```python
from build123d import *

# Parameters (mm, degrees)
F1_DEPTH = 1


with BuildPart() as f1:
    # F0 (on Front) → F1 (new body)
    with BuildSketch(Plane.XZ):
        with BuildLine():
            ThreePointArc((-19.4142135624, 19.4142135624), (-19.847759065, 18.7653668647), (-20, 18))
            Line((-20, 18), (-20, 5))
            ThreePointArc((-20, 5), (-19.7071067812, 4.2928932188), (-19, 4))
            Line((-19, 4), (-16.5, 4))
            ThreePointArc((-16.5, 4), (-15.7928932188, 4.2928932188), (-15.5, 5))
            Line((-15.5, 5), (-15.5, 7))
            ThreePointArc((-15.5, 7), (-15.7928932188, 7.7071067812), (-16.5, 8))
            ThreePointArc((-16.5, 8), (-16.8535533906, 8.1464466094), (-17, 8.5))
            ThreePointArc((-17, 8.5), (-16.4142135624, 9.9142135624), (-15, 10.5))
            Line((-15, 10.5), (-13.0961940777, 10.5))
            ThreePointArc((-13.0961940777, 10.5), (-12.330827213, 10.347759065), (-11.6819805153, 9.9142135624))
            Line((-11.6819805153, 9.9142135624), (-8.3357864376, 6.5680194847))
            ThreePointArc((-8.3357864376, 6.5680194847), (-7.902240935, 5.919172787), (-7.75, 5.1538059223))
            Line((-7.75, 5.1538059223), (-7.75, 0))
            Line((-7.75, 0), (-3.4, 0))
            ThreePointArc((-3.4, 0), (-3.1411904105, 1.30112367), (-2.404163056, 2.404163056))
            Line((-2.404163056, 2.404163056), (-12.2464466094, 12.2464466094))
            ThreePointArc((-12.2464466094, 12.2464466094), (-12.4086582838, 12.1380602337), (-12.6, 12.1))
            Line((-12.6, 12.1), (-17.7, 12.1))
            ThreePointArc((-17.7, 12.1), (-18.0535533906, 12.2464466094), (-18.2, 12.6))
            Line((-18.2, 12.6), (-18.2, 17.2))
            ThreePointArc((-18.2, 17.2), (-18.1238795325, 17.5826834324), (-17.9071067812, 17.9071067812))
            Line((-17.9071067812, 17.9071067812), (-19.4142135624, 19.4142135624))
        make_face()
    extrude(amount=F1_DEPTH)

    # F2: F1 across face


with BuildPart() as f1_1:
    add(f1.part)
    add(f1.part.mirror(Plane(origin=(-7.3253048327, -0.5, 7.3253048327), x_dir=(0, 1, 0), z_dir=(0.7071067812, 0, 0.7071067812))))

    # F3: F1 across face


with BuildPart() as f1_2:
    add(f1_1.part)
    add(f1_1.part.mirror(Plane(origin=(-5.575, -0.5, 0), x_dir=(1, 0, 0), z_dir=(0, 0, -1))))

    # F4: F1 across face


with BuildPart() as f1_3:
    add(f1_2.part)
    add(f1_2.part.mirror(Plane(origin=(0, -0.5, 5.575), x_dir=(0, 1, 0), z_dir=(1, 0, 0))))


solid = f1_3.part
```
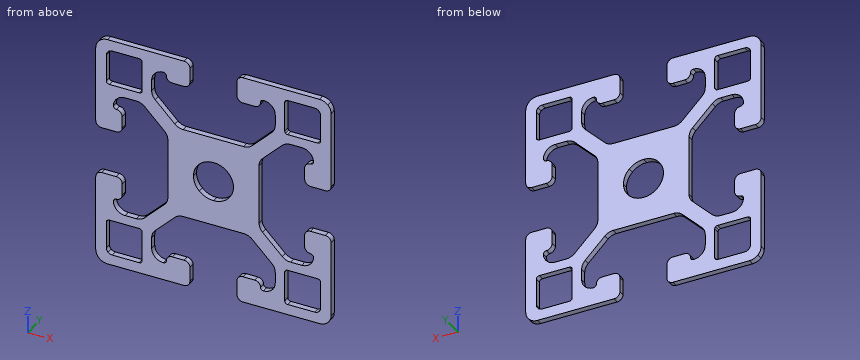
Can you work these out from the model? Positions are in its coordinate system, mm. Coordinates: 2 decimals unless noted, no trailing zeros. Order: outer loops, then holes, each group sorted by start corner. A loop starts at its lowest first (then second) coordinate and runs counter-clockwise, first axis right, second up.
1. If we section it at D-D (y = -0.45): Give the number of separate pieces and of enclosed holes in the cut face, then the cut area to 3 significant figures.
2. If we section it at B-B (x = 1.5): Please give me the cut outline in (y, z), then the cut area to 3 significant figures.
3. If we section it at A-A (x = -14): Please give me the cut outline in (y, z).
4. If we section it at C-C (z = -1.5): Please give me the cut outline in (x, y).
5. I need wall thicknesses on line 1 (X direction, y = -0.3, z = -15); line 2 (X direction, y = -0.55, z = 5); line 3 (Z direction, x = 7.5, y = -0.6). Which ranges of each line are inside material? Lowest first, please.
Entries:
1. separate pieces: 1
1. enclosed holes: 5
1. area: 673 mm2
2. outline: (-1, -7.75) - (0, -7.75) - (0, -3.05) - (-1, -3.05) - close; (-1, 3.05) - (0, 3.05) - (0, 7.75) - (-1, 7.75) - close
2. area: 9.40 mm2
3. outline: (-1, -20) - (0, -20) - (0, -18.2) - (-1, -18.2) - close; (-1, -12.1) - (0, -12.1) - (0, -10.5) - (-1, -10.5) - close; (-1, 10.5) - (0, 10.5) - (0, 12.1) - (-1, 12.1) - close; (-1, 18.2) - (0, 18.2) - (0, 20) - (-1, 20) - close
4. outline: (-7.75, -1) - (-3.05, -1) - (-3.05, 0) - (-7.75, 0) - close; (3.05, -1) - (7.75, -1) - (7.75, 0) - (3.05, 0) - close
5. line 1: x = -20 to -18.2, -12.1 to -10.5, 10.5 to 12.1, 18.2 to 20
5. line 2: x = -20 to -15.5, -7.75 to 7.75, 15.5 to 20
5. line 3: z = -20 to -15.63, -9.27 to 9.27, 15.63 to 20
